Solid Edge part; units mm, degrees
sketch "Sketch1" plane through (0, 0, 0) normal (0, -1, 0) x (1, 0, 0)
  line L0 (-36, 0) -> (0, 0)
  line L1 (0, 0) -> (0, 36)
  line L2 (0, 36) -> (4, 36)
  line L3 (4, 36) -> (4, -4)
  line L4 (4, -4) -> (-36, -4)
  line L5 (-36, -4) -> (-36, 0)
extrude "Protrusion1" add sketch "Sketch1" along normal mid plane 350
sketch "Sketch2" plane through (0, 136, 20) normal (-1, 0, 0) x (0, -1, 0)
  circle A0 centre (172.92, -2) radius 1.6
  circle A1 centre (151, -2) radius 4.5
  circle A2 centre (129.08, -2) radius 1.6
  dimension "D1" = 129.08
extrude "Cutout1" cut sketch "Sketch2" against normal through all
sketch "Sketch3" plane through (0, 136, 18) normal (-1, 0, 0) x (0, -1, 0)
  circle A0 centre (46, 0) radius 4.25
extrude "Cutout2" cut sketch "Sketch3" against normal through all
sketch "Sketch4" plane through (0, 136, 18) normal (-1, 0, 0) x (0, -1, 0)
  circle A0 centre (46, 11) radius 1.6
extrude "Cutout3" cut sketch "Sketch4" against normal through all
pattern_circular "Pattern1" count 4 over 360 about axis through (0, 90, 18) along (1, 0, 0) of "Cutout3"
mirror "Mirror1" about plane through (0, 0, 0) normal (0, -1, 0) of "Cutout2", "Cutout3", "Pattern1"
sketch "Sketch5" plane through (-18, 0, 0) normal (0, 0, 1) x (0, -1, 0)
  circle A0 centre (-155, 2) radius 6.0641
  dimension "D1" = 155
  dimension "D2" = 155
extrude "Cutout4" cut sketch "Sketch5" against normal through all
mirror "Mirror2" about plane through (0, 0, 0) normal (0, -1, 0) of "Cutout4"
properties material "Aluminium, 7075-T6"
Build history of the part. All positions in model axes, mm. A direction names the side the tool comes from. Give positions to 0.01 mm unless a question says otherwise; leave off trailing zeros. Loops run counter-clockwise (first coordinate to the right, second up) from the corner with the lowest first, then second, coordinate; pieces in that order, holes last.
Item 1: Slice it at A-A, the plane y = -15. List the corners of the cut face in (x, z), and give its area (3 significant figures).
Answers follow:
outline: (-36, -4) - (4, -4) - (4, 13.5) - (0, 13.5) - (0, 0) - (-36, 0) - close; (0, 22.5) - (4, 22.5) - (4, 36) - (0, 36) - close
area: 268 mm2
Item 2: Pull direction X, two halves, no side cores. Call faces 3 (the face through (0, 2, 18)), 4 (the face through (1.97, 93.37, 15.41)), 5 (the face through (-19.69, 159.81, -1.97)), 6 (the face through (-12.31, -159.81, -1.97)): released by +X, released by -X, zero draft, split by the parting line, or undercut.
Answers follow:
face 3: released by -X
face 4: zero draft
face 5: undercut
face 6: undercut
Item 3: Drill centre lines: line 1 (Y direction, x = 2, z = 7); line 2 (Z direction, x = 1.55, y = 90); line 3 (X direction, y = -155, z = -2). Where is each one in solid material? Low to high.
Answers follow:
line 1: y = -175 to -91.6, -88.4 to 88.4, 91.6 to 175
line 2: z = -4 to 5.4, 8.6 to 13.75, 22.25 to 27.4, 30.6 to 36
line 3: x = -36 to -22.06, -9.94 to 4
Item 4: Flat gauge pins, fed straight in: pin 1 (10 mm diameter, centred on y = -90, z = 18, fed in from -X); pin 2 (4 mm diameter, centred on y = -90, z = 7, fed in from +X); pin 3 (8 mm diameter, centred on x = -13.5, y = -39, fed in from +Z). Where does each tip first touch, or does it go through?
Answers follow:
pin 1: stops at x = 0
pin 2: stops at x = 4
pin 3: stops at z = 0
Item 5: Slice it at C-C, the plane x = -5. List the corners of the cut face in (y, z).
Answers follow:
outline: (-175, -4) - (175, -4) - (175, 0) - (-175, 0) - close
Item 6: Which spindle directions (+Z, -Z, +X, -X, +Y, -Y) get a long thin tool onto all of the face, cutting with end or side? Do faces 1 (the face through (4, 2, 16)), 2 (the face through (-18, 2, 0)). Say none if no direction does.
Answers follow:
face 1: +Z, -Z, +X, +Y, -Y
face 2: +Z, -X, +Y, -Y
Item 7: Slice it at B-B, the plane y = -154. List the corners of the cut face in (x, z), and give its area (3 significant figures).
Answers follow:
outline: (-36, -4) - (-21.98, -4) - (-21.98, 0) - (-36, 0) - close; (-10.02, -4) - (4, -4) - (4, 36) - (0, 36) - (0, 0) - (-10.02, 0) - close
area: 256 mm2
